The listing builds one solid part. Answer for the finished solid, in the listing's coordinates (mm). Face numbers are marked on the shaded views. A direction names the side the tool comes from. Round coordinates to 2 decimals unless told otherwise and drop trailing zeros. Write each loop counter-clockwise with the first axis right and the second up, starting at its lowest first coordinate (ties: lowest second). Pieces come first, ordered by that corner, then holes.
from build123d import *

# Parameters (mm, degrees)
F0_W     = 25.4
F0_H     = 1219.2
F1_DEPTH = 609.6
F2_W     = 1117.6
F2_H     = 508
F2_W_2   = 1016
F2_H_2   = 406.4
F3_DEPTH = 609.6
F4_W     = 406.4
F4_H     = 406.4
F5_DEPTH = 25.4
F6_W     = 609.6
F6_H     = 25.4
F7_DEPTH = 50.8
F8_W     = 609.6
F8_H     = 25.4
F9_DEPTH = 50.8


with BuildPart() as f1:
    # F0 (on Top) → F1 (new body)
    with BuildSketch(Plane.XY):
        with Locations((12.7, 609.6)):
            Rectangle(F0_W, F0_H)
    extrude(amount=F1_DEPTH)

    # F2 (on face) → F3 (join)
    with BuildSketch(Plane.YZ.offset(25.4)):
        with Locations((609.6, 304.8)):
            Rectangle(F2_W, F2_H)
        with Locations((609.6, 304.8)):
            Rectangle(F2_W_2, F2_H_2, mode=Mode.SUBTRACT)
    extrude(amount=F3_DEPTH)

    # F4 (on face) → F5 (join)
    with BuildSketch(Plane(origin=(0, 0, 0), x_dir=(0, -1, 0), z_dir=(-1, 0, 0))):
        with Locations((-914.4, 304.8)):
            Rectangle(F4_W, F4_H)
        with Locations((-304.8, 304.8)):
            Rectangle(F4_W, F4_H)
    extrude(amount=F5_DEPTH)

    # F6 (on face) → F7 (join)
    with BuildSketch(Plane.XZ.offset(-50.8)):
        with Locations((330.2, 546.1)):
            Rectangle(F6_W, F6_H)
    extrude(amount=F7_DEPTH)

    # F8 (on face) → F9 (join)
    with BuildSketch(Plane(origin=(0, 1168.4, 0), x_dir=(-1, 0, 0), z_dir=(0, 1, 0))):
        with Locations((-330.2, 546.1)):
            Rectangle(F8_W, F8_H)
    extrude(amount=F9_DEPTH)


solid = f1.part
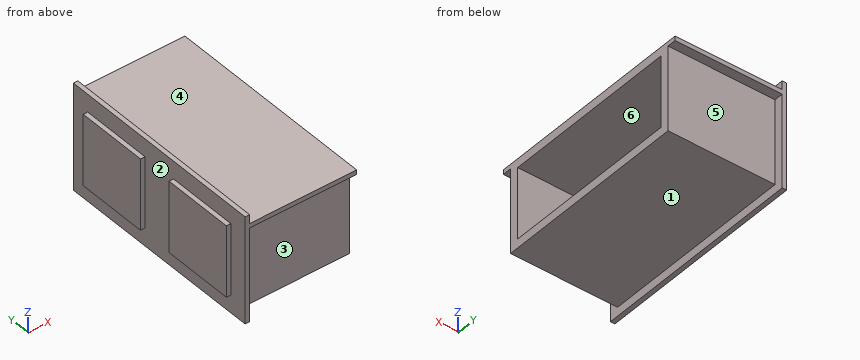
1. Section D-D on y = 940 is taken. Determine the outline of the cut face in (x, z).
Geometry says:
outline: (-25.4, 101.6) - (0, 101.6) - (0, 0) - (25.4, 0) - (25.4, 50.8) - (635, 50.8) - (635, 101.6) - (25.4, 101.6) - (25.4, 508) - (635, 508) - (635, 558.8) - (25.4, 558.8) - (25.4, 609.6) - (0, 609.6) - (0, 508) - (-25.4, 508) - close
2. Given pin 1 (6 mm diameter, centred on x = 295.5, z = 227.5, fed in from +Y); pin 2 (12.5 mm diameter, centred on x = -15, y = 974.5, fed in from +Z); pin 3 (20.5 mm diameter, centred on x = -14, y = 292, fed in from -Z), each flat-ended and moving along its own axis, determine where each tip first touches the part or whether it passes through.
Geometry says:
pin 1: stops at y = 1168.4
pin 2: stops at z = 508
pin 3: stops at z = 101.6
3. Straight lines are drawn through the part: line 1 along Z through (x, y) = (302.5, 189); line 2 along Y through (x, z) = (346.5, 208); line 3 along X through (y, z) = (633.5, 278). For each, find the intervals that lie inside material, in ascending order.
Geometry says:
line 1: z = 50.8 to 101.6, 508 to 558.8
line 2: y = 50.8 to 101.6, 1117.6 to 1168.4
line 3: x = 0 to 25.4
4. Section B-B on z = 289 is taken. Determine the outline of the cut face in (x, y).
Geometry says:
outline: (-25.4, 101.6) - (0, 101.6) - (0, 0) - (25.4, 0) - (25.4, 50.8) - (635, 50.8) - (635, 101.6) - (25.4, 101.6) - (25.4, 1117.6) - (635, 1117.6) - (635, 1168.4) - (25.4, 1168.4) - (25.4, 1219.2) - (0, 1219.2) - (0, 1117.6) - (-25.4, 1117.6) - (-25.4, 711.2) - (0, 711.2) - (0, 508) - (-25.4, 508) - close
5. Section A-A on x = 60 is taken. Determine the outline of the cut face in (y, z).
Geometry says:
outline: (0, 533.4) - (50.8, 533.4) - (50.8, 50.8) - (1168.4, 50.8) - (1168.4, 533.4) - (1219.2, 533.4) - (1219.2, 558.8) - (0, 558.8) - close; hole (101.6, 101.6) - (1117.6, 101.6) - (1117.6, 508) - (101.6, 508) - close
6. A tool of negligible diameter and unlimited length cuts with its end or side. For the marked faces 4, 5 and 6, from which of +Z, -Z, +X, -X, +Y, -Y can it reach the whole face along a straight path? Write none if from no direction.
Geometry says:
face 4: +Z, +X, +Y, -Y
face 5: -Z, +X, +Y
face 6: +X
7. For a pull along Y with two mould halves and no side action, classify the marked faces 1, 2 and 3 as released by +Y, released by -Y, zero draft, split by the parting line, or undercut.
Geometry says:
face 1: zero draft
face 2: undercut
face 3: released by -Y
8. Section C-C on y = 1141.5 is taken. Determine the outline of the cut face in (x, z).
Geometry says:
outline: (0, 0) - (25.4, 0) - (25.4, 50.8) - (635, 50.8) - (635, 558.8) - (25.4, 558.8) - (25.4, 609.6) - (0, 609.6) - close
